Read the model definition and answer for the solid it produces. Units are mm, in the model's axes. A direction names the side the tool comes from. Give positions to 0.01 mm unless a question says otherwise; leave off trailing zeros. Loops run counter-clockwise (first coordinate to the right, second up) from the corner with the lowest first, then second, coordinate; pieces in that order, holes last. Notation, with made-up numbers: (-6.5, -32.5) - (34.5, -32.5) arc R10 cw to (34.5, -20.5) - close; hole circle Ø11 at (-22.5, -2.75). An arc over 180 degrees is marked (long way). Write item = value, one per line.
Solid Edge part; units mm, degrees
sketch "Sketch1" plane through (0, 0, 0) normal (-1, 0, 0) x (0, -1, 0)
  line L0 (2.0853, 0) -> (2.0853, 80)
  line L1 (2.0853, 80) -> (-37.9147, 80)
  line L2 (-37.9147, 80) -> (-37.9147, 0)
  line L3 (-37.9147, 0) -> (2.0853, 0)
extrude "Protrusion1" add sketch "Sketch1" against normal blind 2
sketch "Sketch2" plane through (0, 18.9573, 40) normal (-1, 0, 0) x (0, 0, 1)
  line L0 (-20, 4.9573) -> (-20, 18.9573)
  line L1 (-30, 18.9573) -> (-20, 18.9573)
  line L2 (-30, 18.9573) -> (-30, 4.9573)
  line L3 (-30, 4.9573) -> (-20, 4.9573)
  line L4 (25, 18.9573) -> (25, 4.9573)
  line L5 (25, 4.9573) -> (15, 4.9573)
  line L6 (15, 4.9573) -> (15, 18.9573)
  line L7 (15, 18.9573) -> (25, 18.9573)
extrude "Vysunutí_2" add sketch "Sketch2" along normal blind 3
sketch "Sketch3" plane through (-3, 30.9147, 60) normal (-1, 0, 0) x (0, 0, 1)
  line L0 (5, -17) -> (5, 7)
  line L1 (5, 7) -> (-5, 7)
  line L2 (-5, 7) -> (-5, -17)
  line L3 (-5, -17) -> (5, -17)
  line L4 (-40, -17) -> (-40, 7)
  line L5 (-40, 7) -> (-50, 7)
  line L6 (-50, 7) -> (-50, -17)
  line L7 (-50, -17) -> (-40, -17)
extrude "Vysunutí_3" add sketch "Sketch3" along normal blind 1
sketch "Sketch4" plane through (2, 17.9147, 40) normal (1, 0, 0) x (0, 0, 1)
  line L0 (33, 20) -> (33, -20)
  line L1 (33, -20) -> (35, -20)
  line L2 (35, -20) -> (35, 20)
  line L3 (35, 20) -> (33, 20)
extrude "Protrusion2" add sketch "Sketch4" along normal blind 2
sketch "Sketch5" plane through (2, 17.9147, 36.5) normal (1, 0, 0) x (0, 0, -1)
  line L0 (31.5, 20) -> (31.5, -20)
  line L1 (31.5, -20) -> (33.5, -20)
  line L2 (33.5, -20) -> (33.5, 20)
  line L3 (33.5, 20) -> (31.5, 20)
extrude "Vysunutí_6" add sketch "Sketch5" along normal blind 2
sketch "Sketch6" plane through (2, 17.9147, 39) normal (1, 0, 0) x (0, -1, 0)
  line L0 (19, 39) -> (19, -41)
  line L1 (19, -41) -> (20, -41)
  line L2 (20, -41) -> (20, 39)
  line L3 (20, 39) -> (19, 39)
extrude "Vyříznutí_1" cut sketch "Sketch6" against normal blind 2
sketch "Sketch7" plane through (2, 17.9147, 39) normal (1, 0, 0) x (0, -1, 0)
  line L0 (20, -41) -> (20, 39)
  line L1 (20, 39) -> (19, 39)
  line L2 (19, 39) -> (19, -41)
  line L3 (19, -41) -> (20, -41)
extrude "Vyříznutí_2" cut sketch "Sketch7" along normal blind 2
sketch "Sketch8" plane through (4, 18.4147, 74) normal (1, 0, 0) x (0, -1, 0)
  line L0 (-19.5, -1) -> (-19.5, -1.75)
  line L1 (-19.5, -1.75) -> (19.5, -1.75)
  line L2 (19.5, -1.75) -> (19.5, -1)
  line L3 (19.5, -1) -> (-19.5, -1)
  line L4 (-19.5, 1.75) -> (19.5, 1.75)
  line L5 (19.5, 1.75) -> (19.5, 1)
  line L6 (19.5, 1) -> (-19.5, 1)
  line L7 (-19.5, 1) -> (-19.5, 1.75)
  line L8 (-19.5, 69) -> (-19.5, 68.25)
  line L9 (-19.5, 68.25) -> (19.5, 68.25)
  line L10 (19.5, 68.25) -> (19.5, 69)
  line L11 (19.5, 69) -> (-19.5, 69)
  line L12 (-19.5, 71) -> (-19.5, 71.75)
  line L13 (-19.5, 71.75) -> (19.5, 71.75)
  line L14 (19.5, 71.75) -> (19.5, 71)
  line L15 (19.5, 71) -> (-19.5, 71)
extrude "Protrusion3" add sketch "Sketch8" against normal blind 2
1) The mould has two halves that part along X. Classify faces 1 (the face through (3, 19, 5.75)), 2 (the face through (4, 18, 74)), 3 (the face through (-3, 19, 15)): pulls with the +X half, pulls with the -X half, needs draft (parallel to the pull), parting line crosses it, or undercut.
Output:
face_1 = needs draft
face_2 = pulls with the +X half
face_3 = undercut
2) A cutting plane is placed at D-D on x = -1.5. Determine the outline of the cut face in (y, z), then the cut area to 3 significant figures.
Output:
outline = (23.91, 10) - (37.91, 10) - (37.91, 20) - (23.91, 20) - close; (23.91, 55) - (37.91, 55) - (37.91, 65) - (23.91, 65) - close
area = 280 mm²
3) Find the intervals of material crossed by probe 1 along X at (y, z) = (16.5, 64.5); probe 2 along Z at (x, y) = (2.5, 12); probe 3 along Z at (x, y) = (-1.75, 30), in increasing order.
Output:
probe_1 = -4 to -3, 0 to 2
probe_2 = 2.25 to 5.75, 72.25 to 75.75
probe_3 = 10 to 20, 55 to 65
4) A cutting plane is placed at A-A on x = 2.75. Determine the outline of the cut face in (y, z), then the cut area to 3 significant figures.
Output:
outline = (-1.09, 2.25) - (37.91, 2.25) - (37.91, 5.75) - (-1.09, 5.75) - close; (-1.09, 72.25) - (37.91, 72.25) - (37.91, 75.75) - (-1.09, 75.75) - close
area = 273 mm²
5) A cutting plane is placed at B-B on y = 16.5. Determine the outline of the cut face in (x, z).
Output:
outline = (-4, 10) - (-3, 10) - (-3, 20) - (-4, 20) - close; (-4, 55) - (-3, 55) - (-3, 65) - (-4, 65) - close; (0, 0) - (2, 0) - (2, 2.25) - (4, 2.25) - (4, 5.75) - (2, 5.75) - (2, 72.25) - (4, 72.25) - (4, 75.75) - (2, 75.75) - (2, 80) - (0, 80) - close
6) A tool of negligible diameter and unlimited length cuts with its end or side. For faces 4 (the face through (-2, 29, 55)), 5 (the face through (2, 18, 1)), 6 (the face through (-3, 19, 60)), from which of +Z, -Z, +X, -X, +Y, -Y can it reach the whole face along a straight path? Write none if from no direction.
Output:
face_4 = -X, +Y, -Y
face_5 = -Z, +X, +Y, -Y
face_6 = +Z, -Z, -Y
7) Each of these flat-tipped pins is pushed along its axis until it touches: P1, Ø3, axis at x = -2.5, y = 25.5, coming from the +Z side; P2, Ø1.5, axis at x = -1.5, z = 61, coming from the -Y side; P3, Ø4.5, axis at y = 17, z = 78.5, coming from the +X side. Where does it stop, or does it pass through?
Output:
P1 = 65
P2 = 23.91
P3 = 2
